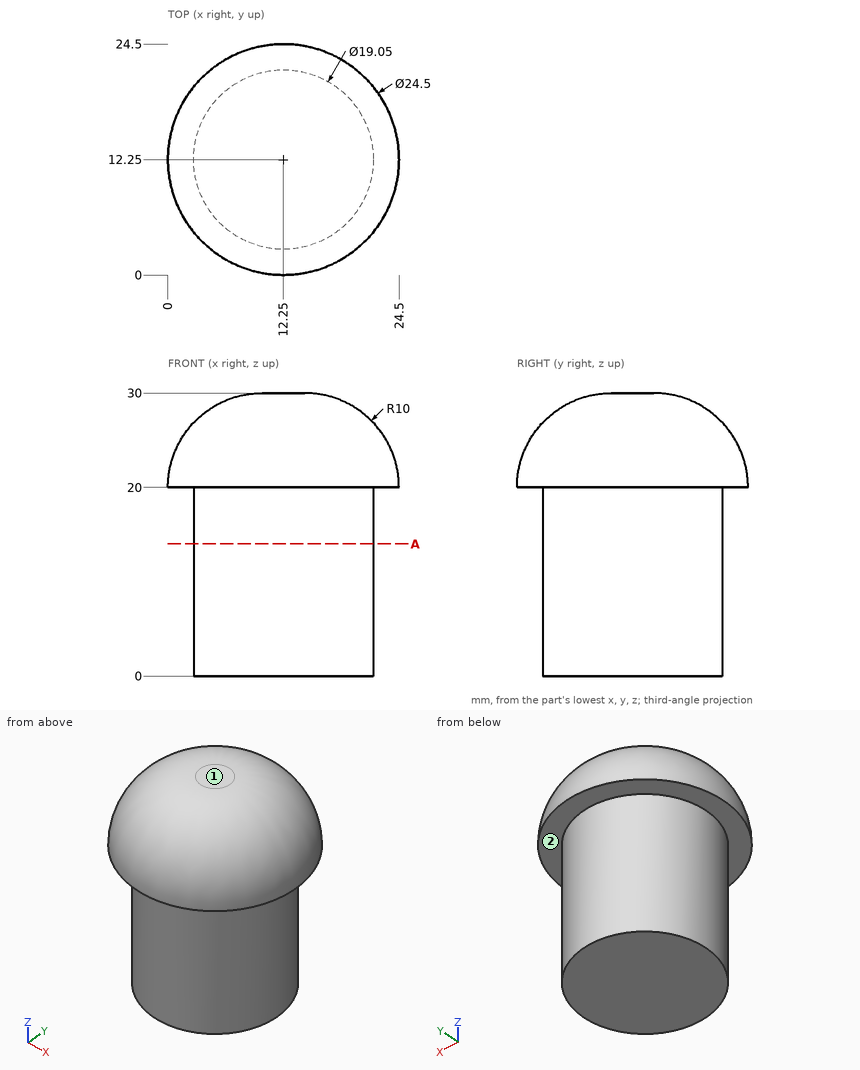
Job drawing, mm, ordinate dimensions from the low corner. One solid piece. A direction names the side the tool comes from. Coordinates: 2 decimals unless noted, no trailing zeros. Loops run counter-clockwise (first coordinate to the right, second up) from the corner with the lowest first, then second, coordinate; pieces in that order, holes last. Notation, with made-up numbers: (74.5, 73.5) -> (131.5, 73.5) arc R30 ccw to (131.5, 101.5) -> close; hole circle Ø11 at (75, 9.25). An arc over 180 degrees is marked (long way). One line per item, written item: value.
1. Which spindle directions (+Z, -Z, +X, -X, +Y, -Y) get a long thin tool onto all of the face, cutting with end or side? Do the marked faces 1 and 2. Say none if no direction does.
Answers:
face 1: +Z, +X, -X, +Y, -Y
face 2: -Z
2. Slice it at A-A on z = 14. Write the cut outline in (x, y) (3 decimals).
Answers:
outline: circle Ø19.05 at (12.25, 12.25)
3. Drill centre lines: line 1 (X direction, y = 12, z = 24.25); line 2 (X direction, y = 9, z = 3); line 3 (Z direction, x = 14.75, y = 5.25). Where is each one in solid material? Low to high. Write a range as [from, to].
Answers:
line 1: x = [0.95, 23.55]
line 2: x = [3.3, 21.2]
line 3: z = [0, 28.55]
4. Flat gauge pins, fed straight in: P1, Ø5, axis at x = 20.5, z = 4, coming from the +Y side; P2, Ø2, axis at x = 10, y = 3.5, coming from the +Z side; P3, Ø6, axis at x = 19.5, z = 8.5, coming from the +Y side. Where does each tip first touch, or does it go through?
Answers:
P1: stops at y = 19.84
P2: stops at z = 28.16
P3: stops at y = 20.77
